Check sheet for the modelled part. Datum: model origin and axes. Units: mm. Face numbers are marked on the shaded views. A direction names the side the tool comes from. Coordinates: 2 decimals unless noted, no trailing zeros. Order: outer loops, then holes, each group sorted by start corner. A loop starts at its lowest first (then second) coordinate and runs counter-clockwise, first axis right, second up.
Autodesk Inventor part; units mm, degrees
ref_plane "YZ Plane" through (0, 0, 0) normal (1, 0, 0) x (0, 1, 0)
ref_plane "XZ Plane" through (0, 0, 0) normal (0, 1, 0) x (-1, 0, 0)
ref_plane "XY Plane" through (0, 0, 0) normal (0, 0, 1) x (1, 0, 0)
sketch "Sketch1" plane through (0, 0, 0) normal (0, 0, 1) x (1, 0, 0)
  circle A0 centre (0, 0) radius 6.35
  circle A1 centre (0, 0) radius 2.3495
  dimension "d0" = 12.7
  dimension "d2" = 4.699
extrude "Extrusion1" add sketch "Sketch1" along normal blind 82.55 contours A0 | A1
extrude "Extrusion2" cut sketch "Sketch1" along normal blind 12.7 contours A1
sketch "Sketch2" plane through (0, 0, 82.55) normal (0, 0, 1) x (1, 0, 0)
  circle A0 centre (0, 0) radius 6.35
  circle A1 centre (0, 0) radius 6
  dimension "d7" = 12
extrude "Extrusion3" add sketch "Sketch2" along normal blind 19.05 contours A1
sketch "Sketch3" plane through (0, 0, 0) normal (0, 0, -1) x (-1, 0, 0)
  circle A0 centre (0, 0) radius 6.35
  line L0 (-1.5875, 6.1484) -> (-1.5875, 4.7625)
  line L1 (-1.5875, 4.7625) -> (1.5875, 4.7625)
  line L2 (1.5875, 4.7625) -> (1.5875, 6.1484)
  line L3 (0, 0) -> (0, 6.35) construction
  point P0 (0, 4.7625)
  dimension "d11" = 3.175
  dimension "d13" = 1.5875
extrude "Extrusion4" cut sketch "Sketch3" against normal blind 79.375 contours L2 L1 L0 A0 picked at (0.1781, 5.2842)
fillet "Fillet1" radius 1.5875 2 edges at (-1.5875, 5.4554, 79.375) (1.5875, 5.4554, 79.375)
chamfer "Chamfer1" distance 0.635 angle 45 2 edges at (5.0201, 3.8886, 0) (-3.8886, -5.0201, 0)
thread "Thread1"
properties part number "P80 Shaft (3.25 inch)" material "Steel"
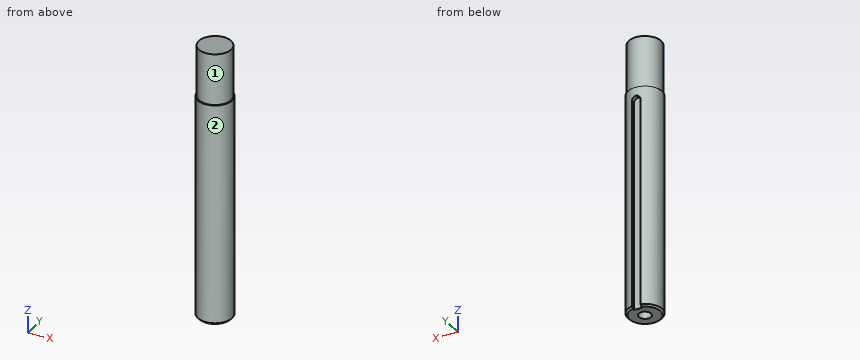
(1) Cross-section at A-A (z = 32.5). Enter the section's corners in (x, y).
Filled in:
outline: (-1.59, 4.76) - (-1.59, 6.15) arc R6.35 ccw (long way) to (1.59, 6.15) - (1.59, 4.76) - close
(2) Tool access check on the marked faces 1 and 2. Record the directions out of +Z, -Z, +X, -X, +Y, -Y that give a thin tool (end or side, any length) a straight path to the whole face; none if there is none.
Filled in:
face 1: +Z
face 2: +Z, -Z
(3) Thickness scan on probe 1 along Y at (x, z) = (0, 9); probe 2 along Z at (x, y) = (1.25, -1.75); probe 3 along X at (y, z) = (-0.25, 95.5). Record the ranges inside material, lowest first.
Filled in:
probe 1: y = -6.35 to -2.35, 2.35 to 4.76
probe 2: z = 12.7 to 101.6
probe 3: x = -5.99 to 5.99
(4) Go/stop test with flat-tipped pins: P1, Ø0.7, axis at y = 5.5, z = 40.5, coming from the -X side; P2, Ø1.1, axis at y = 5, z = 56, coming from the +X side; P3, Ø1.6, axis at x = 0, z = 27, coming from the +Y side. Record where each tip stops, or that it passes through.
Filled in:
P1: stops at x = -3.71
P2: stops at x = 4.53
P3: stops at y = 4.76
